```python
from build123d import *

# Parameters (mm, degrees)
BASPROSKE_W              = 7
BASPROSKE_H              = 23
TOOTHCUT_DEPTH           = 34.271609519
TEETHCUTS_COUNT          = 21
TEETHCUTS_ANGLE          = 342.857142857
HUBNEAONESKE_R           = 5
HUBNEARONE_DEPTH         = 5.0000508
BORSKE_R                 = 3
BORE_DEPTH               = 12.0000508
EXTRUDE_1_DEPTH          = 12.000051
CUT_EXTRUDE_START        = -5.0000508
CUT_EXTRUDE_2_DEPTH      = 5.0000508
CUT_EXTRUDE_3_DEPTH      = 34.250848963
CUT_EXTRUDE_3_DEPTH_BACK = 34.250848963
SKETCH_3_R               = 1.65


with BuildPart() as part:
    # BasProSke → Base-Revolve (revolve)
    with BuildSketch(Plane(origin=(0, 0, 0), x_dir=(1, 0, 0), z_dir=(0, 1, 0)), mode=Mode.PRIVATE) as base_revolve_sk:
        with Locations((3.5, 11.5)):
            Rectangle(BASPROSKE_W, BASPROSKE_H)
    revolve(base_revolve_sk.sketch.rotate(Axis((-10, 0, 0), (1, 0, 0)), 180), axis=Axis((-10, 0, 0), (1, 0, 0)))

    # TooCutSke → ToothCut (cut, through all)
    with BuildSketch(Plane(origin=(0, 0, 0), x_dir=(0, 0, -1), z_dir=(1, 0, 0))):
        with BuildLine():
            ThreePointArc((0.976779145, 18.473194188), (0, 18.499), (-0.976779145, 18.473194188))
            ThreePointArc((-0.976779145, 18.473194188), (-1.625451341, 20.797249275), (-2.90802115, 22.841025768))
            ThreePointArc((-2.90802115, 22.841025768), (0, 23.0254), (2.90802115, 22.841025768))
            ThreePointArc((2.90802115, 22.841025768), (1.625451341, 20.797249275), (0.976779145, 18.473194188))
        make_face()
    toothcut = extrude(amount=TOOTHCUT_DEPTH, mode=Mode.SUBTRACT)

    # TeethCuts: ToothCut ×21 about axis
    teethcuts_axis = Axis((-10, 0, 0), (1, 0, 0))
    for i in range(1, TEETHCUTS_COUNT):
        add(toothcut.rotate(teethcuts_axis, i * TEETHCUTS_ANGLE / (TEETHCUTS_COUNT - 1)), mode=Mode.SUBTRACT)

    # HubNeaOneSke → HubNearOne (add)
    with BuildSketch(Plane.ZY):
        with Locations(Location((0, 0, 0), (0, 0, 180))):
            Circle(HUBNEAONESKE_R)
    extrude(amount=HUBNEARONE_DEPTH)

    # BorSke → Bore (cut, symmetric)
    with BuildSketch(Plane(origin=(0, 0, 0), x_dir=(0, 0, -1), z_dir=(1, 0, 0))):
        with Locations(Location((0, 0, 0), (0, 0, 180))):
            Circle(BORSKE_R)
    extrude(amount=BORE_DEPTH, both=True, mode=Mode.SUBTRACT)

    # 草图1 → 凸台-拉伸1 (add, through all)
    with BuildSketch(Plane.ZY.offset(5.0000508)):
        with BuildLine():
            Line((2.55, 1.580348063), (2.55, -1.580348063))
            ThreePointArc((2.55, -1.580348063), (3, 0), (2.55, 1.580348063))
        make_face()
    extrude(amount=-EXTRUDE_1_DEPTH)

    # 草图4 → 切除-拉伸2 (cut)
    with BuildSketch(Plane.ZY.offset(5.0000508).offset(CUT_EXTRUDE_START)):
        with BuildLine():
            Line((-4, 3), (-4, -3))
            ThreePointArc((-4, -3), (-5, 0), (-4, 3))
        make_face()
        with BuildLine():
            Line((4, 3), (4, -3))
            ThreePointArc((4, -3), (5, 0), (4, 3))
        make_face()
    extrude(amount=CUT_EXTRUDE_2_DEPTH, mode=Mode.SUBTRACT)

    # 草图3 → 切除-拉伸3 (cut, two sides: drawn at the far end of the back side and taken through both)
    with BuildSketch(Plane.XY.offset(-CUT_EXTRUDE_3_DEPTH_BACK)):
        with Locations(Location((-2.5000508, 0, 0), (0, 0, 286.707134567))):
            Circle(SKETCH_3_R)
    extrude(amount=CUT_EXTRUDE_3_DEPTH + CUT_EXTRUDE_3_DEPTH_BACK, mode=Mode.SUBTRACT)


solid = part.part
```
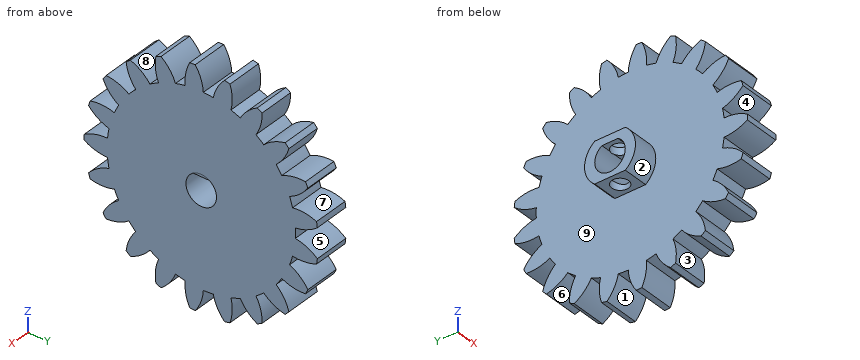
Read the model definition and answer for the solid it produces. Units are mm, in the model's axes. Face numbers are marked on the shaded views. A direction names the side the tool comes from. Coordinates: 2 decimals unless noted, no trailing zeros. Loops run counter-clockwise (first coordinate to the right, second up) from the corner with the lowest first, then second, coordinate; pieces in that order, holes last.
(1) Consider line 1 along Z through (x, y) = (4.25, 15.5); line 2 along X through (y, z) = (9.5, 9.5); line 3 along Z through (x, y) = (0.5, 15). Determine where each line is inside the solid, lowest interval first.
Solution:
line 1: z = -15.78 to -12.01, -10.1 to 10.1, 12.01 to 15.78
line 2: x = 0 to 7
line 3: z = -15.6 to -11.48, -10.83 to 10.83, 11.48 to 15.6
(2) The part is cut by section B-B (y = 4). Determine the outline of the cut face in (x, z).
Solution:
outline: (-5, -3) - (0, -3) - (0, -21.87) - (7, -21.87) - (7, 21.87) - (0, 21.87) - (0, 3) - (-5, 3) - close
(3) The mould has two halves that part along Z. Classify the marked faces 6, 7, 8 and 9: released by +Z, released by -Z, zero draft, split by the parting line, or undercut.
Solution:
face 6: released by -Z
face 7: undercut
face 8: released by +Z
face 9: zero draft
(4) The part is cut by section A-A (z = 0). Determine the outline of the cut face in (x, y), and give its area (3 significant figures).
Solution:
outline: (-5, -5) - (0, -5) - (0, -23) - (7, -23) - (7, -3) - (-5, -3) - close; (-5, 3) - (7, 3) - (7, 18.5) - (0, 18.5) - (0, 5) - (-5, 5) - close
area: 268 mm2
(5) Flat-ended cylindrical pins translate along their axes: pin 1 Ø5 at (x, z) = (-0.5, -1.5) entering from -Y; pin 2 Ø1.6 at (x, y) = (-4, 0.5) entering from -Z; pin 3 Ø1 at (x, y) = (3, 15) entering from -Z; pin 4 Ø4 at (x, z) = (0.5, 16) entering from +Y. Find the tip coordinate at first contact, or state that the pin passes through.
Solution:
pin 1: stops at y = -23
pin 2: stops at z = -4
pin 3: stops at z = -15.78
pin 4: stops at y = 17.23
(6) A tool of negligible diameter and unlimited length cuts with its end or side. For the marked faces 1, 2, 3, 4 and 5, from which of +Z, -Z, +X, -X, +Y, -Y can it reach the whole face along a straight path? Write none if from no direction.
Solution:
face 1: -Z, +X, -X
face 2: -X, -Y
face 3: +X, -X
face 4: +X, -X, -Y
face 5: +X, -X, +Y
